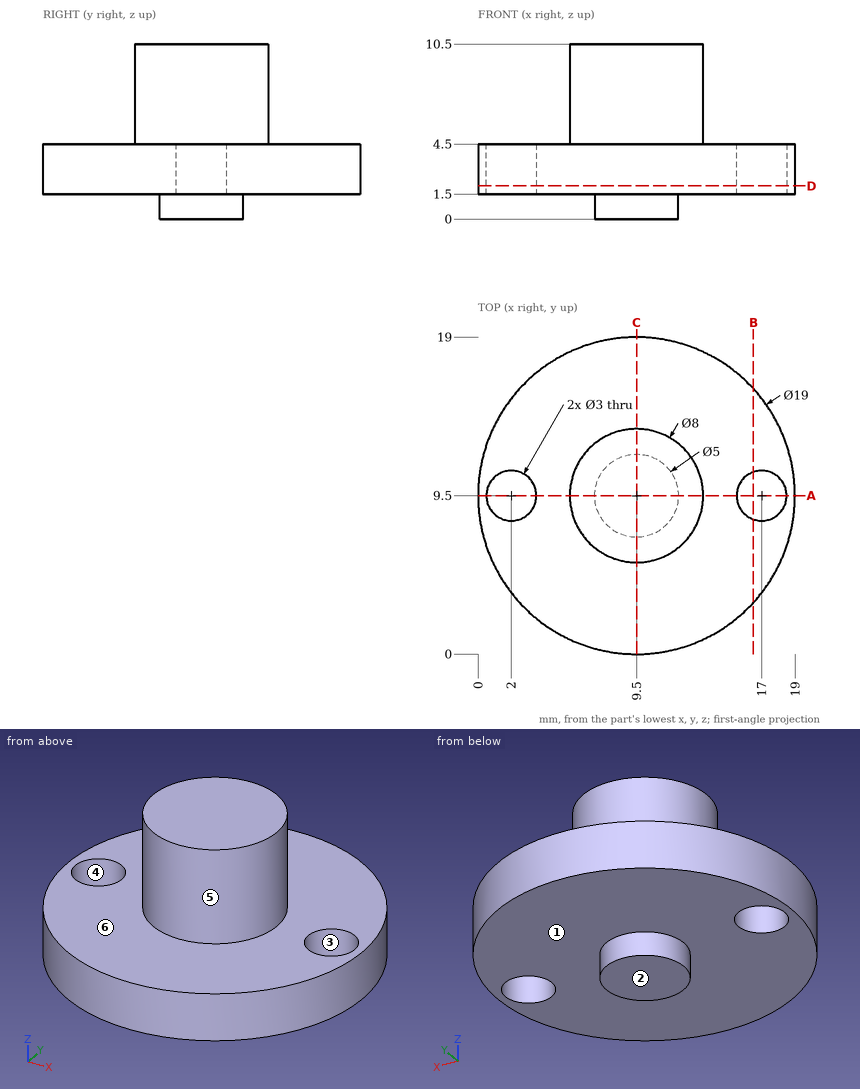
Check sheet for the drawn part. Datum: minimum x, y, z corner. Units: mm. A direction names the side the tool comes from. Coordinates: 2 decimals unless noted, no trailing zeros. Loops run counter-clockwise (first coordinate to the right, second up) from the corner with the lowest first, then second, coordinate; pieces in that order, holes last. Notation, with made-up numbers: M 3,18.25 L 10,18.25 A13 ccw 10,26.25 Z; hole C 14.5,24 d4. An arc over 180 degrees is marked long. Answer as a JSON object with one key per item and string values.
1. Sectioned sample at D-D on z = 2. Record the cut outline in (x, y).
Outcome:
{"outline": "C 9.5,9.5 d19; hole C 2,9.5 d3; hole C 17,9.5 d3"}
2. Sectioned sample at A-A on y = 9.5. Record the cut outline in (x, z).
Outcome:
{"outline": "M 0,1.5 L 0.5,1.5 L 0.5,4.5 L 0,4.5 Z; M 3.5,1.5 L 7,1.5 L 7,0 L 12,0 L 12,1.5 L 15.5,1.5 L 15.5,4.5 L 13.5,4.5 L 13.5,10.5 L 5.5,10.5 L 5.5,4.5 L 3.5,4.5 Z; M 18.5,1.5 L 19,1.5 L 19,4.5 L 18.5,4.5 Z"}
3. Scan lines: L1, parallel to X at y = 10, z = 3.5; L2, parallel to Z at x = 14, y = 9; L3, parallel to Z at x = 6.5, y = 8.25. Record each from-to range of solid material in increasing order. Write a range as from..to.
Outcome:
{"L1": "0.01..0.59, 3.41..15.59, 18.41..18.99", "L2": "1.5..4.5", "L3": "1.5..10.5"}
4. Depth check by flat-ended pin: P1, Ø3, axis at x = 2.5, z = 5, coming from the -Y side; P2, Ø2, axis at y = 11, z = 3.5, coming from the +X side; P3, Ø4, axis at y = 4, z = 9, coming from the -X side; P4, Ø1.8, axis at x = 2, y = 9.5, coming from the -Z side. Enter the tip coordinate at first touch or a pass-through.
Outcome:
{"P1": "y = 1.82", "P2": "x = 18.99", "P3": "x = 7.56", "P4": "through"}
5. Release check for a two-part mould opening along X. For the marked faces 3, 4, 5 and 6 record: pulls with the +X half, pulls with the -X half, needs draft (parallel to the pull), parting line crosses it, or undercut.
Outcome:
{"face 3": "undercut", "face 4": "undercut", "face 5": "parting line crosses it", "face 6": "needs draft"}
6. Access from +Z, -Z, +X, -X, +Y, -Y to the whole of each face (thin tool, end or side, straight path). Record for the marked faces 1 and 2.
Outcome:
{"face 1": "-Z", "face 2": "-Z, +X, -X, +Y, -Y"}
7. Sectioned sample at C-C on x = 9.5. Record the cut outline in (y, z).
Outcome:
{"outline": "M 0,1.5 L 7,1.5 L 7,0 L 12,0 L 12,1.5 L 19,1.5 L 19,4.5 L 13.5,4.5 L 13.5,10.5 L 5.5,10.5 L 5.5,4.5 L 0,4.5 Z"}
8. Sectioned sample at B-B on x = 16.5. Record the cut outline in (y, z).
Outcome:
{"outline": "M 3.08,1.5 L 8.09,1.5 L 8.09,4.5 L 3.08,4.5 Z; M 10.91,1.5 L 15.92,1.5 L 15.92,4.5 L 10.91,4.5 Z"}
